Drawing for the job (mm, zero at the part's lowest x, y, z). Give positions to 0.01 mm unless a question says otherwise; leave off trailing zeros. Order: outer loops, then holes, each group sorted by start corner. A loop starts at its lowest first (then second) coordinate and runs counter-clockwise, first axis right, second up. Notation, with made-up numbers: (42.25, 69.5) - (70.25, 69.5) arc R11 ccw to (70.25, 78.5) - close; hole circle Ø10 at (24, 83). An arc over 180 degrees is marked (long way). One line per item, written item: value.
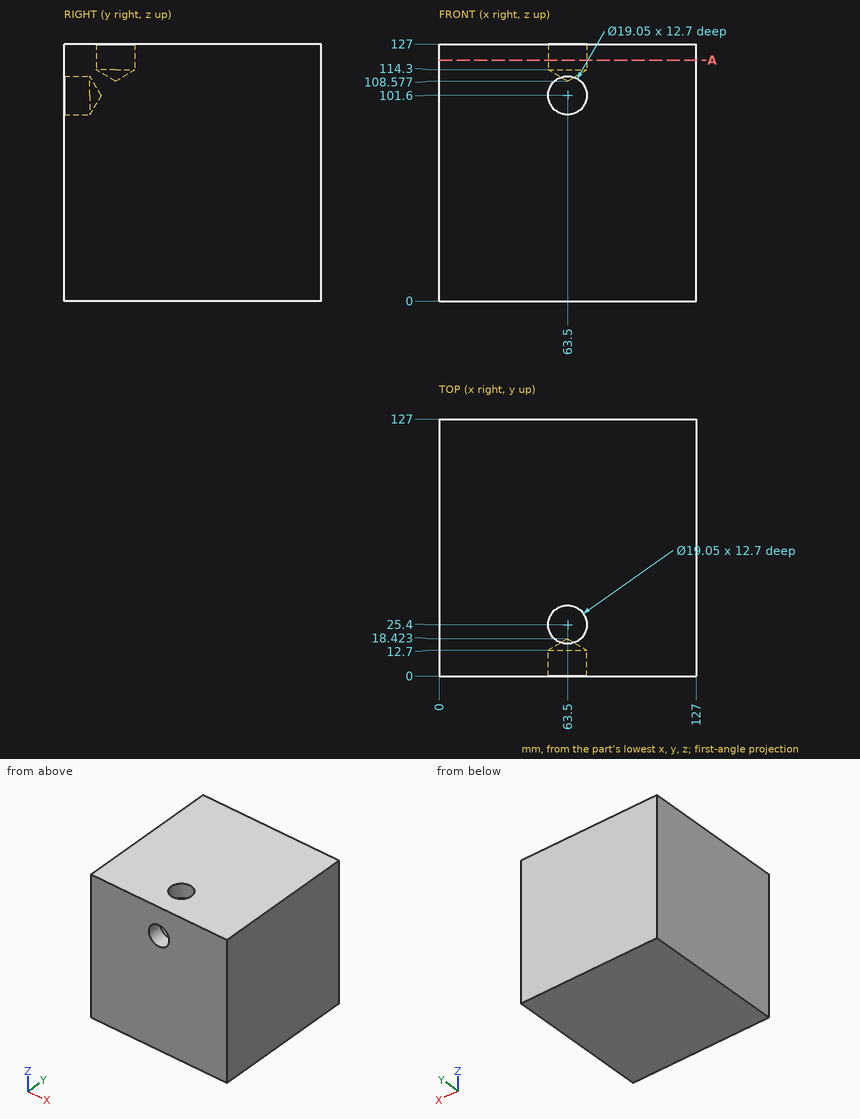
1) Cut at A-A, the plane z = 119. Give the cut face in (x, y) (3 decimals), then the cut area to 3 significant figures.
Outcome:
outline: (0, 0) - (127, 0) - (127, 127) - (0, 127) - close; hole circle Ø19.05 at (63.5, 25.4)
area: 15,800 mm^2
2) Drill centre lines: line 1 along X through (y, z) = (25, 118); line 2 along Y through (x, z) = (63.5, 120.5) (3 decimals); line 3 along Z through (x, y) = (63, 6). Where is each one in solid material? Low to high. Write a range as from..to.
Outcome:
line 1: x = 0..53.98, 73.02..127
line 2: y = 0..15.875, 34.925..127
line 3: z = 0..92.09, 111.11..127
3) Pin check, flat tip, straight feed: pin 1 (11.5 mm diameter, centred on x = 63.5, y = 25.4, fed in from +Z). Stop position of the tip, or through.
Outcome:
pin 1: stops at z = 112.03
